Autodesk Inventor part; units mm, degrees
ref_plane "YZ Plane" through (0, 0, 0) normal (1, 0, 0) x (0, 1, 0)
ref_plane "XZ Plane" through (0, 0, 0) normal (0, 1, 0) x (-1, 0, 0)
ref_plane "XY Plane" through (0, 0, 0) normal (0, 0, 1) x (1, 0, 0)
sketch "Sketch1" plane through (0, 0, 0) normal (0, 1, 0) x (-1, 0, 0)
  line L0 (0, 0) -> (0, -16.256)
  line L1 (0, -16.256) -> (0, -11.811)
  arc A0 (0, -16.256) -> (4.445, -11.811) centre (-0.6095, -11.2015) ccw
  line L2 (0, -16.256) -> (0, -15.3712)
  line L3 (0, -15.3712) -> (0, -14.8015)
  line L4 (4.445, -11.811) -> (4.445, -8.128)
  line L5 (0, 0) -> (0, -2.794)
  line L6 (0, -2.794) -> (4.445, -2.794)
  line L7 (4.445, -2.794) -> (4.445, -8.128)
  line L8 (0, 0) -> (0, -0.508)
  line L9 (4.445, -0.508) -> (4.445, -2.794)
  line L10 (4.445, -0.508) -> (4.191, -0.508)
  line L11 (4.191, -0.508) -> (4.191, 0)
  line L12 (4.191, 0) -> (3.81, 0)
  line L13 (3.81, 0) -> (3.81, -2.794)
  line L14 (4.191, -0.508) -> (4.191, -2.794)
  line L15 (2.0957, -15.5144) -> (2.0957, -11.7468)
  line L16 (2.681, -15.0863) -> (2.681, -11.7468)
  line L17 (2.681, -11.7468) -> (2.0957, -11.7468)
  dimension "d0" = 16.256
  dimension "d2" = 4.445
  dimension "d3" = 2.794
  dimension "d4" = 0.508
  dimension "d5" = 0.254
  dimension "d7" = 0.381
revolve "Revolution1" add sketch "Sketch1" angle 360 about axis through (0, 0, 0) along (0, 0, -1) contours L6 L7 L4 A0 L16 L17 L15 L0 | L13 L12 L11 L14 L6 | L14 L10 L9 L6
sketch "Sketch2" plane through (0, 0, -2.794) normal (0, 0, 1) x (1, 0, 0)
  line L0 (0, 0) -> (0.762, 0)
  line L1 (0.762, 0) -> (0.762, 3.733)
  circle A0 centre (0, 0) radius 3.81
  line L2 (0.762, 0) -> (0.762, -3.733)
  line L3 (0, 0) -> (-0.762, 0)
  line L4 (-0.762, 0) -> (-0.762, 3.733)
  line L5 (-0.762, 0) -> (-0.762, -3.733)
  dimension "d9" = 0.762
  dimension "d10" = 0.762
extrude "Extrusion1" cut sketch "Sketch2" against normal blind 8.89 contours L3 L4 A0 L1 L0 | L0 L2 A0 L5 L3
fillet "Fillet1" radius 1.016 6 edges at (-0.762, -1.8665, -2.794) (-0.762, 1.8665, -2.794) (0.762, 1.8665, -2.794) (0.762, -1.8665, -2.794) (0, 3.81, -11.684) (0, -3.81, -11.684)
properties part number "Pencil Cab"
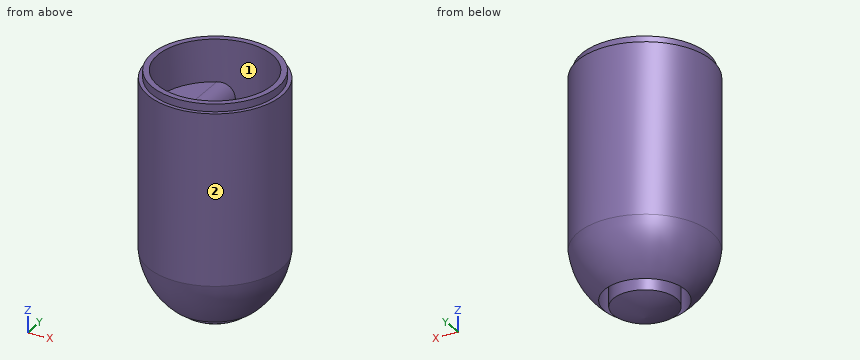
Input: part model. Units: mm. Frame: model coordinates. Face numbers are marked on the shaded views. Give positions to 0.01 mm unless a question says otherwise; leave off trailing zeros. Loops run counter-clockwise (first coordinate to the right, second up) from the corner with the lowest first, then second, coordinate; pieces in that order, holes last. Notation, with made-up numbers: M 48.5,-7.75 L 80.5,-7.75 A25 ccw 80.5,5.25 Z; hole C -10,-16.75 d2. An arc over 180 degrees is marked long. Use CSV: the item, a comma, the result in double quotes.
(1) Pull-direction query (Y, two-part tool) for the marked faces 1 and 2; classes: pulls with the +Y half, pulls with the -Y half, needs draft (parallel to the pull), parting line crosses it, or undercut.
Outcome:
face 1,"undercut"
face 2,"parting line crosses it"
(2) Material intervals for L1, parallel to Y at x = 0, z = -6.5 (3 decimals); L2, parallel to X at y = -0.75, z = -14; L3, parallel to Y at x = 0, z = -12.6, sorted ascending. Write a range as [from, to].
Outcome:
L1,"y = [-4.445, -3.81], [3.81, 4.445]"
L2,"x = [-3.57, -2.57], [-1.96, 1.96], [2.57, 3.57]"
L3,"y = [-4.29, -2.68], [-2.1, 2.1], [2.68, 4.29]"
(3) Section A-A, the plane z = -6. Return loops of the section in (x, y) (3 decimals), plus the area to 3 significant figures.
Outcome:
outline,"C 0,0 d8.89; hole M -0.762,-3.733 A3.81 ccw 0.762,-3.733 L 0.762,3.733 A3.81 ccw -0.762,3.733 Z"
area,"50.5 mm²"
(4) Pin query (flat end, axial travel): P1, Ø2, axis at y = 1.5, z = -6, coming from the +X side; P2, Ø1.6, axis at x = -2.5, y = -0.5, coming from the +Z side; P3, Ø1, axis at x = 3, y = -2, coming from the -Z side; P4, Ø3.5, axis at y = -1, z = -6, coming from the -X side (3 decimals). Return the tip coordinate at first contact, or that it passes through.
Outcome:
P1,"stops at x = 4.42"
P2,"stops at z = -2.79"
P3,"stops at z = -14.68"
P4,"stops at x = -4.445"
